Verification items for this drawing (mm, ordinates from the low corner). A direction names the side the tool comes from. Coordinates: 2 decimals unless noted, no trailing zeros. Order: outer loops, then holes, each group sorted by start corner. A loop starts at its lowest first (then second) coordinate and runs counter-clockwise, first axis right, second up. Notation, with made-up numbers: (44, 83) - (96, 83) arc R18 ccw to (96, 103) - close; hole circle Ø6 at (73.5, -12). An arc over 180 degrees is marked (long way). Use CSV: the item, a comma, the result in double quotes. Start each with the question number.
1) Draft check along X on the marked faces 4, 5, 6 and 7. Enter one of: released by +X, released by -X, zero draft, split by the parting line, or undercut.
2) Sectioned sample at D-D, the plane y = 16.5. Record the cut outline in (x, z), and give its area (3 significant figures).
3) Thickness scan on probe 1 along X at (y, z) = (12.5, 17.5); probe 2 along X at (y, z) = (9.5, 6.5); probe 3 along Z at (x, y) = (11, 16). Record the ranges inside material, lowest first. Write a range as [from, to].
4) Depth check by flat-ended pin: P1, Ø8, axis at x = 37.5, y = 9.5, coming from the +Z side; P2, Ø14, axis at x = 20.5, y = 19, coming from the +Z side; P3, Ø3, axis at x = 13, z = 11.5, coming from the -Y side; P4, Ø8, axis at x = 11.5, z = 20, coming from the +Y side. Enter the tip coordinate at first touch or a pass-through.
5) Sectioned sample at C-C, the plane x = 47. Record the cut outline in (y, z), and give its area (3 significant figures).
6) Sectioned sample at A-A, the plane y = 3.25. Record the cut outline in (x, z), and give its area (3 significant figures).
7) Tool access check on the marked faces 1, 2 and 3. Record the directions out of +Z, -Z, +X, -X, +Y, -Y that give a thin tool (end or side, any length) a straight path to the whole face; none if there is none.
8) Sectioned sample at B-B, the plane z = 2.5. Record the cut outline in (x, y), and give its area (3 significant figures).
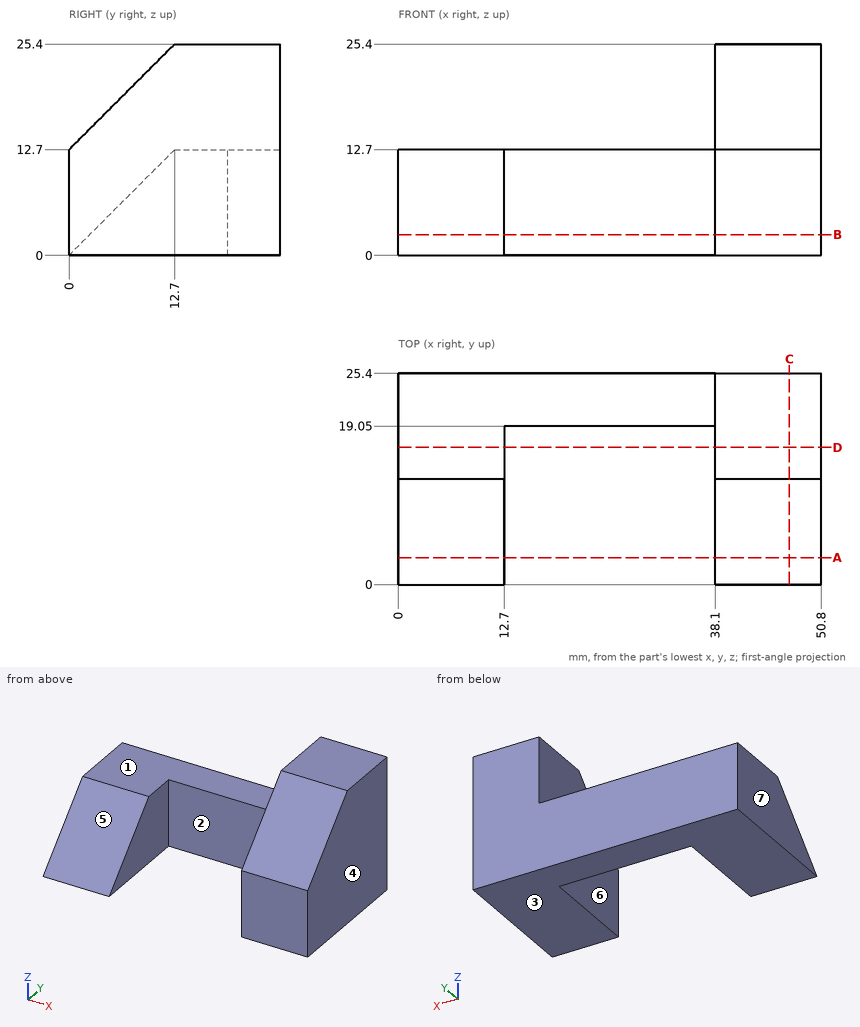
Evaluation:
1,face 4,"released by +X"
1,face 5,"zero draft"
1,face 6,"undercut"
1,face 7,"released by -X"
2,outline,"(0, 0) - (12.7, 0) - (12.7, 12.7) - (0, 12.7) - close; (38.1, 0) - (50.8, 0) - (50.8, 25.4) - (38.1, 25.4) - close"
2,area,"484 mm²"
3,probe 1,"[38.1, 50.8]"
3,probe 2,"[0, 12.7], [38.1, 50.8]"
3,probe 3,"[0, 12.7]"
4,P1,"z = 25.4"
4,P2,"z = 12.7"
4,P3,"y = 10.03"
4,P4,"through"
5,outline,"(0, 0) - (25.4, 0) - (25.4, 25.4) - (12.7, 25.4) - (0, 12.7) - close"
5,area,"565 mm²"
6,outline,"(0, 0) - (12.7, 0) - (12.7, 3.25) - (0, 3.25) - close; (38.1, 0) - (50.8, 0) - (50.8, 15.95) - (38.1, 15.95) - close"
6,area,"244 mm²"
7,face 1,"+Z, -X, +Y, -Y"
7,face 2,"+Z, -Z, -Y"
7,face 3,"-Z, +X, -X, +Y, -Y"
8,outline,"(0, 2.5) - (12.7, 2.5) - (12.7, 19.05) - (38.1, 19.05) - (38.1, 0) - (50.8, 0) - (50.8, 25.4) - (0, 25.4) - close"
8,area,"775 mm²"
